Part model, mm, in its own coordinate system. Face numbers are marked on the shaded views. A direction names the side the tool comes from. Give positions to 0.01 mm unless a question says otherwise; leave off trailing zeros. Order: outer loops, then holes, each group sorted by start corner. A loop starts at its lowest first (then second) coordinate and runs counter-clockwise, first axis right, second up. Notation, with made-up numbers: M 7,16 L 17,16 A23 ccw 17,24 Z; hole C -27,-23.75 d8. An arc over 180 degrees is marked long. Return JSON: item names as keys, results as strings.
from build123d import *

# Parameters (mm, degrees)
SKETCH_1_W          = 71
SKETCH_1_H          = 39
EXTRUDE_1_DEPTH     = 24
EXTRUDE_2_DEPTH     = 2
SKETCH_3_W          = 67
SKETCH_3_H          = 32
CUT_EXTRUDE_1_DEPTH = 1


with BuildPart() as part:
    # 草图1 → 凸台-拉伸1 (new body)
    with BuildSketch(Plane.XY):
        Rectangle(SKETCH_1_W, SKETCH_1_H)
    extrude(amount=EXTRUDE_1_DEPTH)

    # 草图2 → 凸台-拉伸2 (add)
    with BuildSketch(Plane.XY.offset(24)):
        with BuildLine():
            Line((-37.5, -21.5), (37.5, -21.5))
            ThreePointArc((37.5, -21.5), (38.914213562, -20.914213562), (39.5, -19.5))
            Line((39.5, -19.5), (39.5, 19.5))
            ThreePointArc((39.5, 19.5), (38.914213562, 20.914213562), (37.5, 21.5))
            Line((37.5, 21.5), (-37.5, 21.5))
            ThreePointArc((-37.5, 21.5), (-38.914213562, 20.914213562), (-39.5, 19.5))
            Line((-39.5, 19.5), (-39.5, -19.5))
            ThreePointArc((-39.5, -19.5), (-38.914213562, -20.914213562), (-37.5, -21.5))
        make_face()
    extrude(amount=EXTRUDE_2_DEPTH)

    # 草图3 → 切除-拉伸1 (cut)
    with BuildSketch(Plane.XY.offset(26)):
        Rectangle(SKETCH_3_W, SKETCH_3_H)
    extrude(amount=-CUT_EXTRUDE_1_DEPTH, mode=Mode.SUBTRACT)


solid = part.part
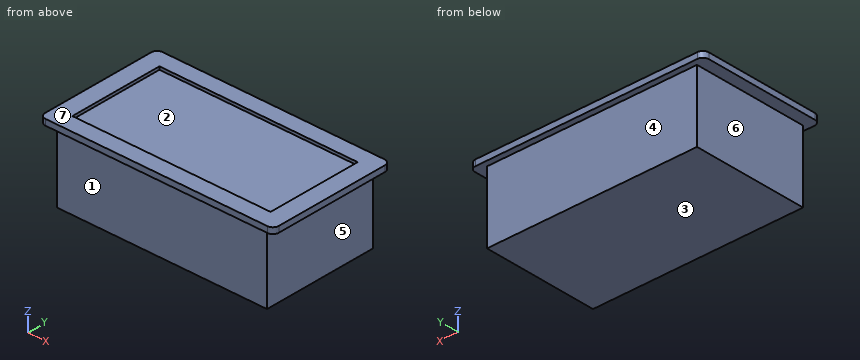
Q1. Probe line 1 along Y through (x, z) = (-6, 16); line 2 along Z through (x, y) = (-14.5, 5); line 3 along X through (y, z) = (-8, 22). List the from-to ranges inside material, lowest first.
Established:
{"line 1": "y = -19.5 to 19.5", "line 2": "z = 0 to 25", "line 3": "x = -35.5 to 35.5"}
Q2. Band-saw the part on D-D (y = -14). Give the cut face in (x, z).
Established:
{"outline": "M -39.5,24 L -35.5,24 L -35.5,0 L 35.5,0 L 35.5,24 L 39.5,24 L 39.5,26 L 33.5,26 L 33.5,25 L -33.5,25 L -33.5,26 L -39.5,26 Z"}
Q3. Band-saw the part on B-B (x = 9). Give the cut face in (y, z).
Established:
{"outline": "M -21.5,24 L -19.5,24 L -19.5,0 L 19.5,0 L 19.5,24 L 21.5,24 L 21.5,26 L 16,26 L 16,25 L -16,25 L -16,26 L -21.5,26 Z"}
Q4. Band-saw the part on C-C (z = 10.75). Give the cut face in (x, y).
Established:
{"outline": "M -35.5,-19.5 L 35.5,-19.5 L 35.5,19.5 L -35.5,19.5 Z"}
Q5. Pin check, flat tips, straight feed: pin 1 (4 mm diameter, centred on x = 29, z = 6.5, fed in from -Y); pin 2 (1 mm diameter, centred on y = 14.5, z = 17.5, fed in from +X); pin 3 (2 mm diameter, centred on y = 5.5, z = 18, fed in from -X). Stop position of each tip, or through.
Established:
{"pin 1": "stops at y = -19.5", "pin 2": "stops at x = 35.5", "pin 3": "stops at x = -35.5"}
Q6. Band-saw the part on A-A (y = 18). Give the cut face in (x, z), then the cut area to 3 significant figures.
Established:
{"outline": "M -39.5,24 L -35.5,24 L -35.5,0 L 35.5,0 L 35.5,24 L 39.5,24 L 39.5,26 L -39.5,26 Z", "area": "1,860 mm²"}
Q7. 3-axis set-ups, long thin cutter, end or side, ignore diameter. For the marked faces 5, 6 and 7: which of +Z, -Z, +X, -X, +Y, -Y reach the whole face in a straight line?
Established:
{"face 5": "-Z, +X, +Y, -Y", "face 6": "-Z, -X, +Y, -Y", "face 7": "+Z, +X, -X, +Y, -Y"}
Q8. Two-plate mould, pull along Y, no slides. Class the marked faces 1, 2, 3 and 4: +Y half, -Y half, draft (parallel to the pull), parting line (faces both ways), or undercut.
Established:
{"face 1": "-Y half", "face 2": "undercut", "face 3": "draft", "face 4": "+Y half"}
